Input: part model. Units: mm. Frame: model coordinates. A direction names the side the tool comes from. Give positions to 0.01 mm unless a question says otherwise; leave off trailing zeros. Loops run counter-clockwise (first coordinate to the right, second up) from the corner with the lowest first, then second, coordinate; pieces in that order, holes last. Notation, with made-up numbers: (-23, 58.25) -> (-4, 58.25) arc R23 cw to (-4, 67.25) -> close; hole circle Ø1 at (64, -14.75). An arc over 180 degrees is marked (long way). Use CSV: the item, a comma, the result in double quotes.
```python
from build123d import *

# Parameters (mm, degrees)
RESSALTO_EXTRUS_O1_DEPTH = 13
RESSALTO_EXTRUS_O2_DEPTH = 3


with BuildPart() as part:
    # Esboço1 → Ressalto-extrusão1 (new body)
    with BuildSketch(Plane.XY):
        with BuildLine():
            Line((-111.248828562, 3.491171507), (-12.504488884, 3.410248792))
            Line((-12.504488884, 3.410248792), (-12.46323751, 53.746420916))
            ThreePointArc((-12.46323751, 53.746420916), (-12.930939325, 54.878175435), (-14.061925745, 55.347731606))
            Line((-14.061925745, 55.347731606), (-109.606266497, 55.426031866))
            ThreePointArc((-109.606266497, 55.426031866), (-110.738021017, 54.958330051), (-111.207577187, 53.82734363))
            Line((-111.207577187, 53.82734363), (-111.248828562, 3.491171507))
        make_face()
        Polygon((-108.746780608, 5.989121875), (-15.002439252, 5.912296746), (-14.963974236, 52.848470011), (-108.708315592, 52.92529514), align=None, mode=Mode.SUBTRACT)
    extrude(amount=RESSALTO_EXTRUS_O1_DEPTH)

    # Esboço2 → Ressalto-extrusão2 (add)
    with BuildSketch(Plane(origin=(0, 0, 0), x_dir=(-1, 0, 0), z_dir=(0, 0, -1))):
        with BuildLine():
            Line((9.463238518, 53.743962364), (9.506948443, 0.407791248))
            Line((9.506948443, 0.407791248), (114.251286106, 0.493631066))
            Line((114.251286106, 0.493631066), (114.20757618, 53.829802182))
            ThreePointArc((114.20757618, 53.829802182), (112.857602189, 57.081388141), (109.603807945, 58.426030858))
            Line((109.603807945, 58.426030858), (14.059467194, 58.347730599))
            ThreePointArc((14.059467194, 58.347730599), (10.807881235, 56.997756608), (9.463238518, 53.743962364))
        make_face()
    extrude(amount=RESSALTO_EXTRUS_O2_DEPTH)


solid = part.part
```
1) Mould query, pull axis Y, two halves, no side actions, for faces 3 (the cylindrical face through (-112.89, 57.05, -1.48)), 4 (the flat face through (-61, 30, 0)), 5 (the flat face through (-66, 4, 13)). Classes: pulls with the +Y half, pulls with the -Y half, needs draft (parallel to the pull), parting line crosses it, or undercut.
From the geometry:
face 3,"pulls with the +Y half"
face 4,"undercut"
face 5,"needs draft"
2) Section query B-B (x = -86.5). Return loops of the section in (y, z).
From the geometry:
outline,"(0.47, -3) -> (58.41, -3) -> (58.41, 0) -> (55.41, 0) -> (55.41, 13) -> (52.91, 13) -> (52.91, 0) -> (5.97, 0) -> (5.97, 13) -> (3.47, 13) -> (3.47, 0) -> (0.47, 0) -> close"
3) Section query C-C (y = 41.5). Return loops of the section in (x, z), then the cut area to 3 significant figures.
From the geometry:
outline,"(-114.22, -3) -> (-9.47, -3) -> (-9.47, 0) -> (-12.47, 0) -> (-12.47, 13) -> (-14.97, 13) -> (-14.97, 0) -> (-108.72, 0) -> (-108.72, 13) -> (-111.22, 13) -> (-111.22, 0) -> (-114.22, 0) -> close"
area,"379 mm^2"
4) Section query A-A (z = 8). Return loops of the section in (x, y), then the cut area to 3 significant figures.
From the geometry:
outline,"(-111.25, 3.49) -> (-12.5, 3.41) -> (-12.46, 53.75) arc R1.6 ccw to (-14.06, 55.35) -> (-109.61, 55.43) arc R1.6 ccw to (-111.21, 53.83) -> close; hole (-108.75, 5.99) -> (-15, 5.91) -> (-14.96, 52.85) -> (-108.71, 52.93) -> close"
area,"727 mm^2"
5) Contact query for flat-ended pins moving along their axis: pin 1 (12 mm diameter, centred on x = -43.5, y = 19, fed in from +Z); pin 2 (1 mm diameter, centred on y = 35.5, z = 0, fed in from -X); pin 3 (3 mm diameter, centred on x = -66.5, z = 3, fed in from -Y). Output: stop coordinate, or through.
From the geometry:
pin 1,"stops at z = 0"
pin 2,"stops at x = -114.22"
pin 3,"stops at y = 3.45"
6) Ray query, line 1 (X direction, y = 33.5, z = 3.25); line 2 (Y direction, x = -82, z = 10.5); line 3 (Y direction, x = -34, z = 10.25). Return the intervals inside material, ascending.
From the geometry:
line 1,"x = -111.22 to -108.72, -14.98 to -12.48"
line 2,"y = 3.47 to 5.97, 52.9 to 55.4"
line 3,"y = 3.43 to 5.93, 52.86 to 55.36"
7) Reachability of faces 1 (the flat face through (-61, 30, -3)), 2 (the flat face through (-62, 2, 0)) from +Z, -Z, +X, -X, +Y, -Y: full face, straight path, thin tool, end or side. Return the list, or none.
From the geometry:
face 1,"-Z, +X, -X, +Y, -Y"
face 2,"+Z"
